from build123d import *

# Parameters (mm, degrees)
ESQUISSE1_W             = 20
ESQUISSE1_H             = 15
BOSS_EXTRU_3_DEPTH      = 1
ESQUISSE1_5_W           = 10
ESQUISSE1_5_H           = 5
BOSS_EXTRU_4_DEPTH      = 2
ESQUISSE1_6_W           = 4
ESQUISSE1_6_H           = 5
BOSS_EXTRU_5_DEPTH      = 15
BOSS_EXTRU_6_DEPTH      = 3
ESQUISSE1_8_W           = 7
ESQUISSE1_8_H           = 2
ESQUISSE1_8_R           = 0.15
BOSS_EXTRU_7_DEPTH      = 1
BOSS_EXTRU_7_DEPTH_BACK = 4
ESQUISSE1_9_R           = 0.15
BOSS_EXTRU_8_DEPTH      = 8


with BuildPart() as part:
    # Esquisse1 → Boss.-Extru.3 (new body)
    with BuildSketch(Plane(origin=(0, 0, 0), x_dir=(1, 0, 0), z_dir=(0, 1, 0))):
        with Locations((-29.903190877, 15.678459307)):
            Rectangle(ESQUISSE1_W, ESQUISSE1_H)
    extrude(amount=-BOSS_EXTRU_3_DEPTH)

    # Esquisse1_5 → Boss.-Extru.4 (add)
    with BuildSketch(Plane(origin=(0, 0, 0), x_dir=(1, 0, 0), z_dir=(0, 1, 0))):
        with Locations((-29.903190877, 12.678459307)):
            Rectangle(ESQUISSE1_5_W, ESQUISSE1_5_H)
    extrude(amount=BOSS_EXTRU_4_DEPTH)

    # Esquisse1_6 → Boss.-Extru.5 (add)
    with BuildSketch(Plane(origin=(0, 0, 0), x_dir=(1, 0, 0), z_dir=(0, 1, 0))):
        with Locations((-36.903190877, 12.678459307)):
            Rectangle(ESQUISSE1_6_W, ESQUISSE1_6_H)
        with Locations((-22.903190877, 12.678459307)):
            Rectangle(ESQUISSE1_6_W, ESQUISSE1_6_H)
    extrude(amount=BOSS_EXTRU_5_DEPTH)

    # Esquisse1_7 → Boss.-Extru.6 (add)
    with BuildSketch(Plane(origin=(0, 0, 0), x_dir=(1, 0, 0), z_dir=(0, 1, 0))):
        with BuildLine():
            ThreePointArc((-25.903190877, 18.178459307), (-24.903190877, 17.178459307), (-25.903190877, 16.178459307))
            Line((-25.903190877, 16.178459307), (-33.903190877, 16.178459307))
            ThreePointArc((-33.903190877, 16.178459307), (-34.903190877, 17.178459307), (-33.903190877, 18.178459307))
            Line((-33.903190877, 18.178459307), (-25.903190877, 18.178459307))
        make_face()
    extrude(amount=BOSS_EXTRU_6_DEPTH)

    # Esquisse1_8 → Boss.-Extru.7 (add, two sides)
    with BuildSketch(Plane(origin=(0, 0, 0), x_dir=(1, 0, 0), z_dir=(0, 1, 0))) as boss_extru_7_sk:
        with Locations((-29.903190877, 21.405559188)):
            Rectangle(ESQUISSE1_8_W, ESQUISSE1_8_H)
        with Locations((-27.903190877, 21.405559188)):
            Circle(ESQUISSE1_8_R, mode=Mode.SUBTRACT)
        with Locations((-29.903190877, 21.405559188)):
            Circle(ESQUISSE1_8_R, mode=Mode.SUBTRACT)
        with Locations((-31.903190877, 21.405559188)):
            Circle(ESQUISSE1_8_R, mode=Mode.SUBTRACT)
    extrude(amount=BOSS_EXTRU_7_DEPTH)
    extrude(boss_extru_7_sk.sketch, amount=-BOSS_EXTRU_7_DEPTH_BACK)

    # Esquisse1_9 → Boss.-Extru.8 (add)
    with BuildSketch(Plane(origin=(0, 0, 0), x_dir=(1, 0, 0), z_dir=(0, 1, 0))):
        with Locations((-31.903190877, 21.405559188)):
            Circle(ESQUISSE1_9_R)
        with Locations((-29.903190877, 21.405559188)):
            Circle(ESQUISSE1_9_R)
        with Locations((-27.903190877, 21.405559188)):
            Circle(ESQUISSE1_9_R)
    extrude(amount=-BOSS_EXTRU_8_DEPTH)


solid = part.part
Verification items for the finished model (mm, model axes). A direction names the side the tool comes from. Coordinates: 2 decimals unless noted, no trailing zeros. Order: outer loops, then holes, each group sorted by start corner. A loop starts at its lowest first (then second) coordinate and runs counter-clockwise, first axis right, second up.
Item 1: Section check A-A, the plane y = 4. Enter the section's corners in (x, z), then the cut area to 3 significant figures.
Filled in:
outline: (-38.9, -15.18) - (-34.9, -15.18) - (-34.9, -10.18) - (-38.9, -10.18) - close; (-24.9, -15.18) - (-20.9, -15.18) - (-20.9, -10.18) - (-24.9, -10.18) - close
area: 40.0 mm2
Item 2: Access from +Z, -Z, +X, -X, +Y, -Y to the whole of each face (thin tool, end or side, straight path). Record for faces 4 (the face through (-30, 1, -18.178)), 5 (the face through (-20.903, 7, -13)), 6 (the face through (-30, -2, -20.406)).
Filled in:
face 4: +X, -X, +Y
face 5: +Z, -Z, +X, +Y
face 6: +Z, +X, -X, -Y
Item 3: Release check for a two-part mould opening along X. For faces 1 (the face through (-33.403, 0.5, -21.4)), 2 (the face through (-19.903, -0.5, -15.6)), 3 (the face through (-30, 2, -13)) record: +X half, -X half, draft (parallel to the pull), parting line (faces both ways), or undercut.
Filled in:
face 1: -X half
face 2: +X half
face 3: undercut
Item 4: Section check D-D, the plane y = -4.75. Enter the section's corners in (x, z), then the cut area to 3 significant figures.
Filled in:
outline: circle Ø0.3 at (-31.9, -21.41); circle Ø0.3 at (-29.9, -21.41); circle Ø0.3 at (-27.9, -21.41)
area: 0.212 mm2
Item 5: Material ranges on L1, parallel to X at y = 11.5, z = -13.5; L2, parallel to Y at x = -27, z = -10.75; L3, parallel to Y at x = -21.25, z = -15.75, recorded low to high.
Filled in:
L1: x = -38.9 to -34.9, -24.9 to -20.9
L2: y = -1 to 2
L3: y = -1 to 0
Item 6: Depth check by flat-ended pin: pin 1 (2.5 mm diameter, centred on y = 9.5, z = -12.5, fed in from -X); pin 2 (4 mm diameter, centred on x = -37.5, z = -17, fed in from -Y); pin 3 (1.5 mm diameter, centred on x = -30, y = -3, fed in from -Z). Enter the tip coordinate at first touch or a pass-through.
Filled in:
pin 1: stops at x = -38.9
pin 2: stops at y = -1
pin 3: stops at z = -22.41
Item 7: Section check B-B, the plane x = -37. Enter the section's corners in (y, z), then the cut area to 3 significant figures.
Filled in:
outline: (-1, -23.18) - (0, -23.18) - (0, -15.18) - (15, -15.18) - (15, -10.18) - (0, -10.18) - (0, -8.18) - (-1, -8.18) - close
area: 90.0 mm2
Item 8: Section check C-C, the plane z = -13.5. Enter the section's corners in (x, y), then the cut area to 3 significant figures.
Filled in:
outline: (-39.9, -1) - (-19.9, -1) - (-19.9, 0) - (-20.9, 0) - (-20.9, 15) - (-24.9, 15) - (-24.9, 2) - (-34.9, 2) - (-34.9, 15) - (-38.9, 15) - (-38.9, 0) - (-39.9, 0) - close
area: 160 mm2
